```python
from build123d import *

# Parameters (mm, degrees)
ESQUISSE1_R                         = 11.1
ESQUISSE1_R_2                       = 1.65
ESQUISSE1_R_3                       = 2.5
ESQUISSE1_W                         = 4.6
ESQUISSE1_H                         = 8.6
ESQUISSE1_W_2                       = 8.6
ESQUISSE1_H_2                       = 4.6
BOSS_EXTRU_1_DEPTH                  = 13
CHANFREIN1_SIZE                     = 2
ENL_V_MAT_EXTRU_1_REACH             = 55.956
ESQUISSE2_R                         = 2.65
ENL_V_MAT_EXTRU_1_DIRECTION_2_DEPTH = 54.955560846
R_P_TITION_CIRCULAIRE1_COUNT        = 4


with BuildPart() as part:
    # Esquisse1 → Boss.-Extru.1 (new body)
    with BuildSketch(Plane.XY):
        with BuildLine():
            Line((-23.741352507, -6.2), (-23.741352507, 6.2))
            Line((-23.741352507, 6.2), (-29.147898724, 6.2))
            ThreePointArc((-29.147898724, 6.2), (-21.071782079, 21.071782079), (-6.2, 29.147898724))
            Line((-6.2, 29.147898724), (-6.2, 23.741352507))
            Line((-6.2, 23.741352507), (6.2, 23.741352507))
            Line((6.2, 23.741352507), (6.2, 29.147898724))
            ThreePointArc((6.2, 29.147898724), (21.071782079, 21.071782079), (29.147898724, 6.2))
            Line((29.147898724, 6.2), (23.741352507, 6.2))
            Line((23.741352507, 6.2), (23.741352507, -6.2))
            Line((23.741352507, -6.2), (29.147898724, -6.2))
            ThreePointArc((29.147898724, -6.2), (21.071782079, -21.071782079), (6.2, -29.147898724))
            Line((6.2, -29.147898724), (6.2, -23.741352507))
            Line((6.2, -23.741352507), (-6.2, -23.741352507))
            Line((-6.2, -23.741352507), (-6.2, -29.147898724))
            ThreePointArc((-6.2, -29.147898724), (-21.071782079, -21.071782079), (-29.147898724, -6.2))
            Line((-29.147898724, -6.2), (-23.741352507, -6.2))
        make_face()
        with Locations(Location((0, 0, 0), (0, 0, 180))):
            Circle(ESQUISSE1_R, mode=Mode.SUBTRACT)
        with Locations(Location((-15.5, 15.5, 0), (0, 0, 180))):
            Circle(ESQUISSE1_R_2, mode=Mode.SUBTRACT)
        with Locations(Location((15.5, 15.5, 0), (0, 0, 180))):
            Circle(ESQUISSE1_R_2, mode=Mode.SUBTRACT)
        with Locations(Location((15.5, -15.5, 0), (0, 0, 180))):
            Circle(ESQUISSE1_R_2, mode=Mode.SUBTRACT)
        with Locations(Location((-15.5, -15.5, 0), (0, 0, 180))):
            Circle(ESQUISSE1_R_2, mode=Mode.SUBTRACT)
        with Locations(Location((-8.029746973, 17.219847954, 0), (0, 0, 180))):
            Circle(ESQUISSE1_R_3, mode=Mode.SUBTRACT)
        with Locations(Location((8.029746973, 17.219847954, 0), (0, 0, 180))):
            Circle(ESQUISSE1_R_3, mode=Mode.SUBTRACT)
        with Locations(Location((17.219847954, 8.029746973, 0), (0, 0, 180))):
            Circle(ESQUISSE1_R_3, mode=Mode.SUBTRACT)
        with Locations(Location((17.219847954, -8.029746973, 0), (0, 0, 180))):
            Circle(ESQUISSE1_R_3, mode=Mode.SUBTRACT)
        with Locations(Location((8.029746973, -17.219847954, 0), (0, 0, 180))):
            Circle(ESQUISSE1_R_3, mode=Mode.SUBTRACT)
        with Locations(Location((-8.029746973, -17.219847954, 0), (0, 0, 180))):
            Circle(ESQUISSE1_R_3, mode=Mode.SUBTRACT)
        with Locations(Location((-17.219847954, -8.029746973, 0), (0, 0, 180))):
            Circle(ESQUISSE1_R_3, mode=Mode.SUBTRACT)
        with Locations(Location((-17.219847954, 8.029746973, 0), (0, 0, 180))):
            Circle(ESQUISSE1_R_3, mode=Mode.SUBTRACT)
        with Locations((-16.656153343, 0.3)):
            Rectangle(ESQUISSE1_W, ESQUISSE1_H, mode=Mode.SUBTRACT)
        with Locations((0.106768766, 16.462922109)):
            Rectangle(ESQUISSE1_W_2, ESQUISSE1_H_2, mode=Mode.SUBTRACT)
        with Locations((16.269690876, -0.3)):
            Rectangle(ESQUISSE1_W, ESQUISSE1_H, mode=Mode.SUBTRACT)
        with Locations((-0.493231234, -16.462922109)):
            Rectangle(ESQUISSE1_W_2, ESQUISSE1_H_2, mode=Mode.SUBTRACT)
    extrude(amount=BOSS_EXTRU_1_DEPTH)

    # Chanfrein1
    chanfrein1_edges = [part.edges().sort_by_distance(p)[0] for p in [
        (-13.85, 15.5, 13),
        (17.15, 15.5, 13),
        (17.15, -15.5, 13),
        (-13.85, -15.5, 13),
    ]]
    chamfer(chanfrein1_edges, length=CHANFREIN1_SIZE)

    # Esquisse2 → Enlèv. mat.-Extru.1 (cut, up to next)
    with BuildSketch(Plane.ZY.offset(14.356153343), mode=Mode.PRIVATE) as enl_v_mat_extru_1_sk1:
        with Locations(Location((7, 0, 0), (0, 0, 180))):
            Circle(ESQUISSE2_R)
    enl_v_mat_extru_1_tool1 = extrude(enl_v_mat_extru_1_sk1.sketch, amount=-ENL_V_MAT_EXTRU_1_REACH, mode=Mode.PRIVATE) & part.part
    enl_v_mat_extru_1 = enl_v_mat_extru_1_tool1.solids().sort_by_distance((-14.356153, 0, 7))[0]
    add(enl_v_mat_extru_1, mode=Mode.SUBTRACT)

    # Esquisse2 → Enlèv. mat.-Extru.1 direction 2 (cut)
    with BuildSketch(Plane.ZY.offset(14.356153343)):
        with Locations(Location((7, 0, 0), (0, 0, 180))):
            Circle(ESQUISSE2_R)
    enl_v_mat_extru_1_direction_2 = extrude(amount=ENL_V_MAT_EXTRU_1_DIRECTION_2_DEPTH, mode=Mode.SUBTRACT)

    # Répétition circulaire1: Enlèv. mat.-Extru.1, Enlèv. mat.-Extru.1 direction 2 ×4 about axis
    r_p_tition_circulaire1_axis = Axis((0, 0, 0), (0, 0, -1))
    add([enl_v_mat_extru_1.rotate(r_p_tition_circulaire1_axis, i * 360 / R_P_TITION_CIRCULAIRE1_COUNT) for i in range(1, R_P_TITION_CIRCULAIRE1_COUNT)], mode=Mode.SUBTRACT)
    add([enl_v_mat_extru_1_direction_2.rotate(r_p_tition_circulaire1_axis, i * 360 / R_P_TITION_CIRCULAIRE1_COUNT) for i in range(1, R_P_TITION_CIRCULAIRE1_COUNT)], mode=Mode.SUBTRACT)


solid = part.part
```
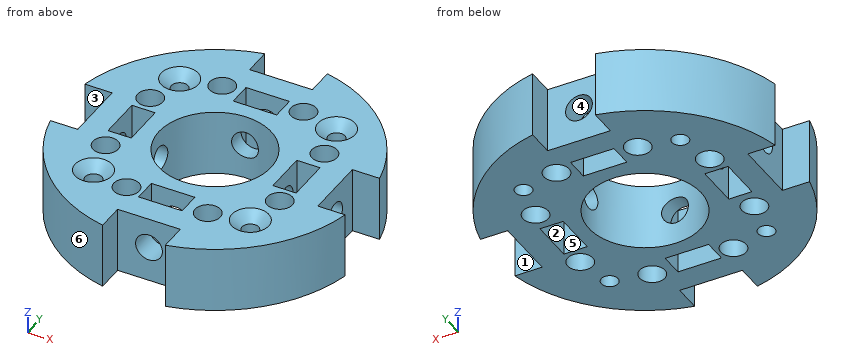
Geometry check sheet. Reference: the model listing, model coordinates, mm. Face numbers are marked on the shaded views. A direction names the side the tool comes from. Round coordinates to 2 decimals unless told otherwise and drop trailing zeros. Order: outer loops, then holes, each group sorted by start corner. A loop starts at its lowest first (then second) coordinate and runs counter-clockwise, first axis right, second up. Notation, with made-up numbers: M 60.5,53 L 81.5,53 A15 ccw 81.5,64 Z; hole C 10,36 d10. An arc over 180 degrees is marked long. Answer as CSV lines item,"result".
1) Mould release check, pull along Y, two halves, no side actions. Record for the marked faces 4, 5 and 6: +Y half, -Y half, draft (parallel to the pull), parting line (faces both ways), or undercut.
Entries:
face 4,"draft"
face 5,"undercut"
face 6,"-Y half"
2) Thickness scan on probe 1 along Y at (x, z) = (0, 3); probe 2 along X at (y, z) = (16.5, 5.5); probe 3 along Y at (x, z) = (18, 5). Record the ranges inside material, lowest first. Write a range as [from, to].
Entries:
probe 1,"[-23.74, -18.76], [-14.16, -11.1], [11.1, 14.16], [18.76, 23.74]"
probe 2,"[-24.82, -16.81], [-14.19, -10.42], [-5.64, -4.19], [4.41, 5.64], [10.42, 14.19], [16.81, 24.82]"
probe 3,"[-23.75, -10.4], [-5.65, -4.6], [4, 5.65], [10.4, 23.75]"
3) Gauge pin test, flat ends, axial feed: pin 1 Ø2.5 at (x, z) = (0, 9.5) entering from -Y; pin 2 Ø4.5 at (y, z) = (-0.5, 6.5) entering from -X; pin 3 Ø1.4 at (y, z) = (-15.5, 7) entering from -X. Record the tip position at first contact, or that the pin passes through.
Entries:
pin 1,"y = -23.74"
pin 2,"x = -23.74"
pin 3,"x = -25.87"
4) Tool access check on the marked faces 1, 2 and 3. Record the directions out of +Z, -Z, +X, -X, +Y, -Y that give a thin tool (end or side, any length) a straight path to the whole face; none if there is none.
Entries:
face 1,"+Z, -Z, +X"
face 2,"+Z, -Z"
face 3,"+Z, -Z, -X"
5) Sectioned sample at C-C on y = 7. Record the cut outline in (x, z), and give its area (3 significant figures).
Entries:
outline,"M -28.97,0 L -19.5,0 L -19.5,13 L -28.97,13 Z; M -14.94,0 L -8.61,0 L -8.61,13 L -14.94,13 Z; M 8.61,0 L 14.94,0 L 14.94,13 L 8.61,13 Z; M 19.5,0 L 28.97,0 L 28.97,13 L 19.5,13 Z"
area,"411 mm2"
6) Sectioned sample at A-A on x = 0. Give the number of separate pieces and of enclosed holes in the cut face, and give its area (3 significant figures).
Entries:
separate pieces,"8"
enclosed holes,"0"
area,"124 mm2"
